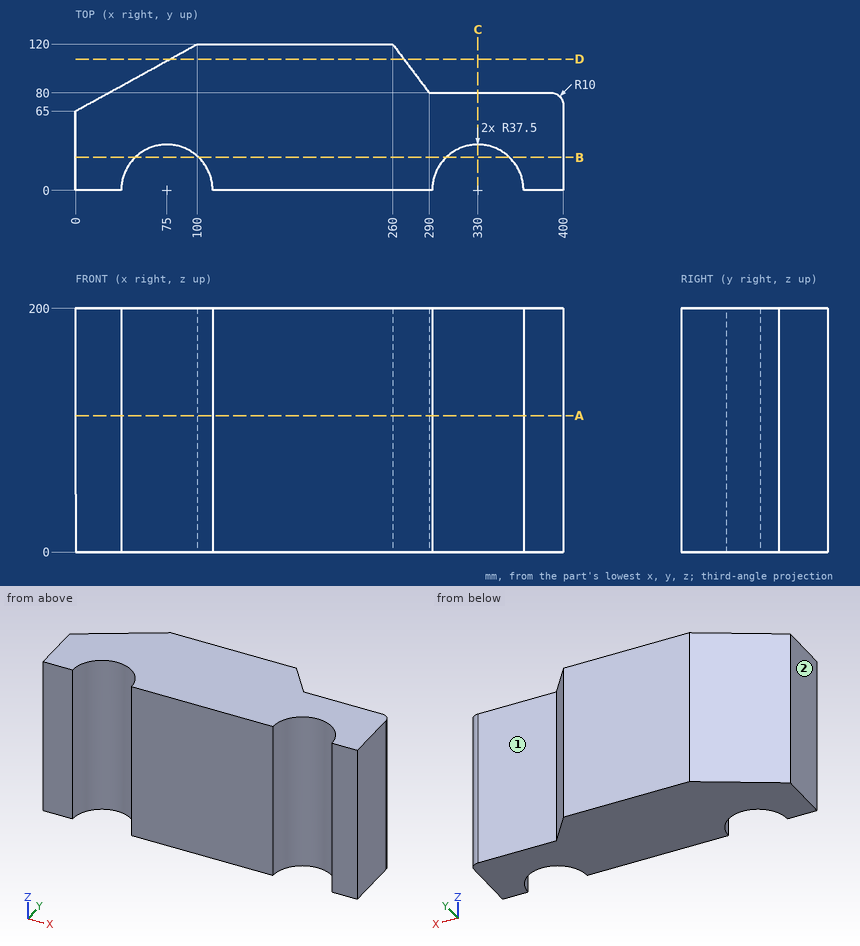
Job drawing, mm, ordinate dimensions from the low corner. One solid piece. A direction names the side the tool comes from. Round coordinates to 2 decimals unless told otherwise and drop trailing zeros. Loops run counter-clockwise (first coordinate to the right, second up) from the corner with the lowest first, then second, coordinate; pieces in that order, holes last.
(1) Cut at A-A (z = 112). Give the cut face in (x, y), plus the area to 3 significant figures.
(2) Cut at D-D (y = 107.5). Give the cut face in (x, z) (3 decimals).
(3) Cut at C-C (x = 330). Give the cut face in (y, z), plus the area to 3 significant figures.
(4) Which spindle directions (+Z, -Z, +X, -X, +Y, -Y) get a long thin tool onto all of the face, cutting with end or side? Do the marked faces 1 and 2. Say none if no direction does.
(5) Cut at B-B (y = 27). Give the cut face in (x, z).
(6) Drop flat-ended pins along their axis: pin 1 (5 mm diameter, centred on x = 200, z = 126, fed in from -Y); pin 2 (1 mm diameter, centred on x = 101.5, z = 46.5, fed in from -Y); pin 3 (1 mm diameter, centred on x = 61, z = 34, fed in from -Y). Give the stop position or say it passes through.
(7) Wall check: line 1 along X through (y, z) = (16.5, 185); line 2 along X through (y, z) = (28, 174.5); line 3 along Y through (x, z) = (372, 151.5). Give the ranges that are in metal, low to high.
Findings below:
1. outline: (0, 0) - (37.5, 0) arc R37.5 cw to (112.5, 0) - (292.5, 0) arc R37.5 cw to (367.5, 0) - (400, 0) - (400, 70) arc R10 ccw to (390, 80) - (290, 80) - (260, 120) - (100, 120) - (0, 65) - close
1. area: 35,800 mm2
2. outline: (77.273, 0) - (269.375, 0) - (269.375, 200) - (77.273, 200) - close
3. outline: (37.5, 0) - (80, 0) - (80, 200) - (37.5, 200) - close
3. area: 8,500 mm2
4. face 1: +Z, -Z, +X, +Y
4. face 2: +Z, -Z, -X, +Y, -Y
5. outline: (0, 0) - (48.98, 0) - (48.98, 200) - (0, 200) - close; (101.02, 0) - (303.98, 0) - (303.98, 200) - (101.02, 200) - close; (356.02, 0) - (400, 0) - (400, 200) - (356.02, 200) - close
6. pin 1: stops at y = 0
6. pin 2: stops at y = 26.02
6. pin 3: stops at y = 34.58
7. line 1: x = 0 to 41.33, 108.67 to 296.33, 363.67 to 400
7. line 2: x = 0 to 50.06, 99.94 to 305.06, 354.94 to 400
7. line 3: y = 0 to 80
